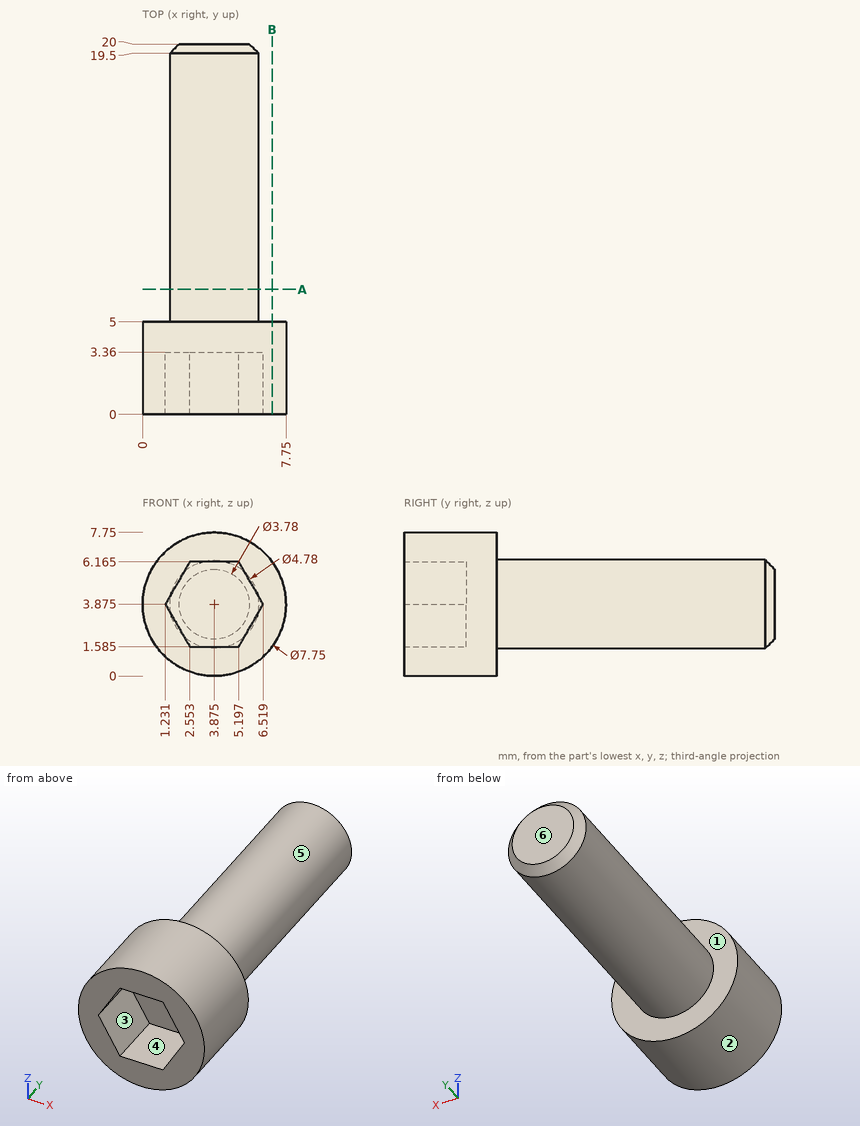
Design review of the part shown in the three views and the two pictorial views. Dimensions are in mm from the part's minimum x, y and z. A direction names the side the tool comes from. Round coordinates to 2 decimals unless told otherwise and drop trailing zeros. Loops run counter-clockwise (first coordinate to the right, second up) from the corner with the lowest first, then second, coordinate; pieces in that order, holes last. Notation, with made-up numbers: (87.25, 31.5) - (111.25, 31.5) arc R9 cw to (111.25, 41.5) - close; hole circle Ø9 at (-16, 60). An arc over 180 degrees is marked (long way). One line per item, written item: value. Start each with the question number.
Item 1: Take a section at B-B (x = 7). Give the boundary of the cut face in (y, z), plus the area to 3 significant figures.
Item 2: For the marked faces 4, 5 and 6, list the 3-axis set-ups (+Z, -Z, +X, -X, +Y, -Y) from which the entire face can be reached by the end or side of a thin tool; tool diameter is ignored.
Item 3: Take a section at A-A (y = 6.75). Give the boundary of the cut face in (x, z) (1 decimal).
Item 4: For L1, parallel to Y at x = 4, z = 7; L2, parallel to Z at x = 3.75, y = 5.75, list the stretches that pass through material, from the lowest coordinate up.
Item 5: Clearance check with flat-ended pins moving along their axes: pin 1 Ø1 at (x, y) = (2, 16.5) entering from -Z; pin 2 Ø0.8 at (x, y) = (3.5, 1.5) entering from -Z; pin 3 Ø1.4 at (x, z) = (3.5, 4.5) entering from -Y; pin 4 Ø1 at (x, z) = (7, 2) entering from +Y. State where each tip first meets the part, or that it passes through.
Item 6: The part is to be moulded in two halves that separate along X. For the marked faces 1, 2 and 3, say which applies: +X half, -X half, draft (parallel to the pull), parting line (faces both ways), or undercut.
Answer below:
1. outline: (0, 1.58) - (5, 1.58) - (5, 6.17) - (0, 6.17) - close
1. area: 22.9 mm2
2. face 4: -Y
2. face 5: +Y
2. face 6: +Z, -Z, +X, -X, +Y
3. outline: circle Ø4.8 at (3.9, 3.9)
4. L1: y = 0 to 5
4. L2: z = 1.49 to 6.26
5. pin 1: stops at z = 1.92
5. pin 2: stops at z = 0
5. pin 3: stops at y = 3.36
5. pin 4: stops at y = 5
6. face 1: draft
6. face 2: parting line
6. face 3: undercut
